Geometry: see drawing. Coordinates: mm, zero at the bounding-box minimum. A direction names the side the tool comes from. Coordinates: 2 decimals unless noted, no trailing zeros. Write each loop counter-clockwise with the first axis right and the second up, starting at its lowest first coordinate (ties: lowest second). Pieces come first, ordered by that corner, then holes. Notation, with made-up numbers: M 54.5,-15.5 L 98.5,-15.5 A23 cw 98.5,2.5 Z; hole C -4,35 d2. An arc over 180 degrees is marked long. Answer as CSV lines item,"result". Start each with the question number.
1. Section B-B on y = 3.75. Return the cut outline in (x, z).
2. Reachability of the marked faces 1 and 2 from +Z, -Z, +X, -X, +Y, -Y: full face, straight path, thin tool, end or side. Return the list, or none.
3. Line query: probe 1 along X at (y, z) = (7.75, 31.5); probe 2 along Z at (x, y) = (12, 2.5); probe 3 along Z at (x, y) = (18, 2). Output: solid intervals per line, ascending. Write a range as [from, to].
4. Section D-D on x = 34.5. Return the cut outline in (y, z).
5. Contact query for flat-ended pins moving along their axis: pin 1 Ø0.5 at (x, z) = (32, 30.5) entering from -Y; pin 2 Ø0.6 at (y, z) = (7.5, 30.5) entering from -X; pin 3 Ø6.5 at (x, y) = (20.5, 9.5) entering from +Z. Output: stop coordinate, or through.
6. Section A-A on z = 16. Return the cut outline in (x, y), plus the area to 3 significant figures.
7. Mould query, pull axis X, two halves, no side actions, for the marked faces 3, 4 and 5. Classes: pulls with the +X half, pulls with the -X half, needs draft (parallel to the pull), parting line crosses it, or undercut.
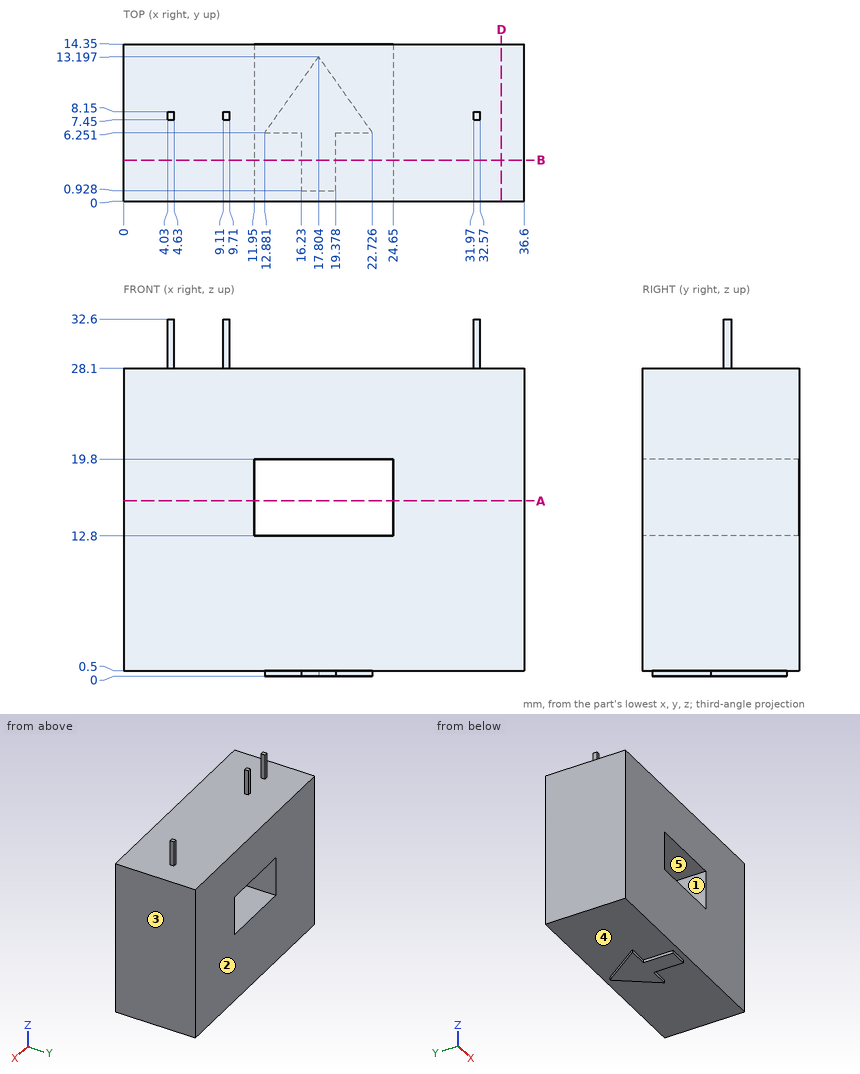
Values:
1,outline,"M 0,0.5 L 16.23,0.5 L 16.23,0 L 19.38,0 L 19.38,0.5 L 36.6,0.5 L 36.6,28.1 L 0,28.1 Z; hole M 11.95,12.8 L 24.65,12.8 L 24.65,19.8 L 11.95,19.8 Z"
2,face 1,"+Y, -Y"
2,face 2,"+Z, -Z, +X, -X, +Y"
3,probe 1,"[4.03, 4.63], [9.11, 9.71], [31.97, 32.57]"
3,probe 2,"[0.5, 12.8], [19.8, 28.1]"
3,probe 3,"[0, 12.8], [19.8, 28.1]"
4,outline,"M 0,0.5 L 14.35,0.5 L 14.35,28.1 L 0,28.1 Z"
5,pin 1,"y = 7.45"
5,pin 2,"x = 4.03"
5,pin 3,"z = 28.1"
6,outline,"M 0,0 L 11.95,0 L 11.95,14.35 L 0,14.35 Z; M 24.65,0 L 36.6,0 L 36.6,14.35 L 24.65,14.35 Z"
6,area,"343 mm²"
7,face 3,"pulls with the +X half"
7,face 4,"needs draft"
7,face 5,"undercut"
